Verification items for this drawing (mm, ordinates from the low corner). A direction names the side the tool comes from. Round coordinates to 2 decimals unless told otherwise and drop trailing zeros. Order: outer loops, then holes, each group sorted by start corner. A loop starts at its lowest first (then second) coordinate and runs counter-clockwise, first axis right, second up. Notation, with made-up numbers: (74.25, 12) - (94.25, 12) arc R17 cw to (94.25, 30) - close; hole circle Ø4 at (61.25, 45). An arc over 180 degrees is marked (long way). One line per question, with ' | ' between items. Start each with the question number.
Q1. Sectioned sample at A-A, the plane y = 6. Enter the section's corners in (x, z).
Q2. Gauge pin test, flat ends, axial feed: P1, Ø2, axis at y = 24, z = 1.5, coming from the -X side; P2, Ø0.6, axis at y = 6.5, z = 3, coming from the -X side; P3, Ø0.8, axis at x = 10.5, y = 5, coming from the +Z side; P4, Ø0.8, axis at x = 2, y = 4.5, coming from the -Z side. Record the tip position at first contact, or that the pin passes through.
Q3. Sectioned sample at B-B, the plane x = 5.5. Enter the section's corners in (y, z).
Q4. Sectioned sample at C-C, the plane z = 1. Enter the section's corners in (x, y), then the cut area to 3 significant figures.
Q5. Material ranges on line 1 along Y through (x, z) = (5.75, 2.5), recorded low to high.
Q6. Tool access check on the marked faces 1, 2 and 3. Record the directions out of +Z, -Z, +X, -X, +Y, -Y that give a thin tool (end or side, any length) a straight path to the whole face; none if there is none.
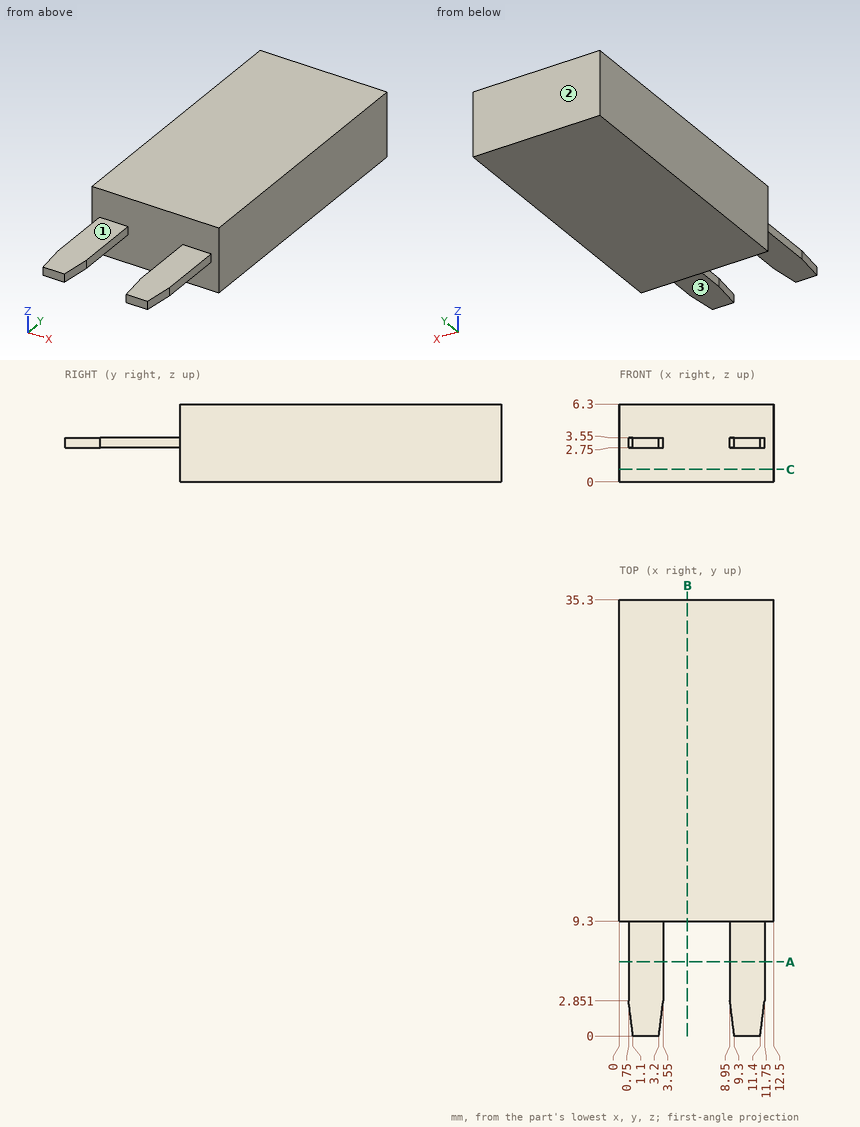
Determined:
1) outline: (0.75, 2.75) - (3.55, 2.75) - (3.55, 3.55) - (0.75, 3.55) - close; (8.95, 2.75) - (11.75, 2.75) - (11.75, 3.55) - (8.95, 3.55) - close
2) P1: stops at x = 0 | P2: stops at x = 0.75 | P3: stops at z = 3.55 | P4: stops at z = 2.75
3) outline: (9.3, 0) - (35.3, 0) - (35.3, 6.3) - (9.3, 6.3) - close
4) outline: (0, 9.3) - (12.5, 9.3) - (12.5, 35.3) - (0, 35.3) - close | area: 325 mm2
5) line 1: y = 9.3 to 35.3
6) face 1: +Z, +X, -X, -Y | face 2: +Z, -Z, +X, -X, +Y | face 3: -Z, +X, -X, -Y
